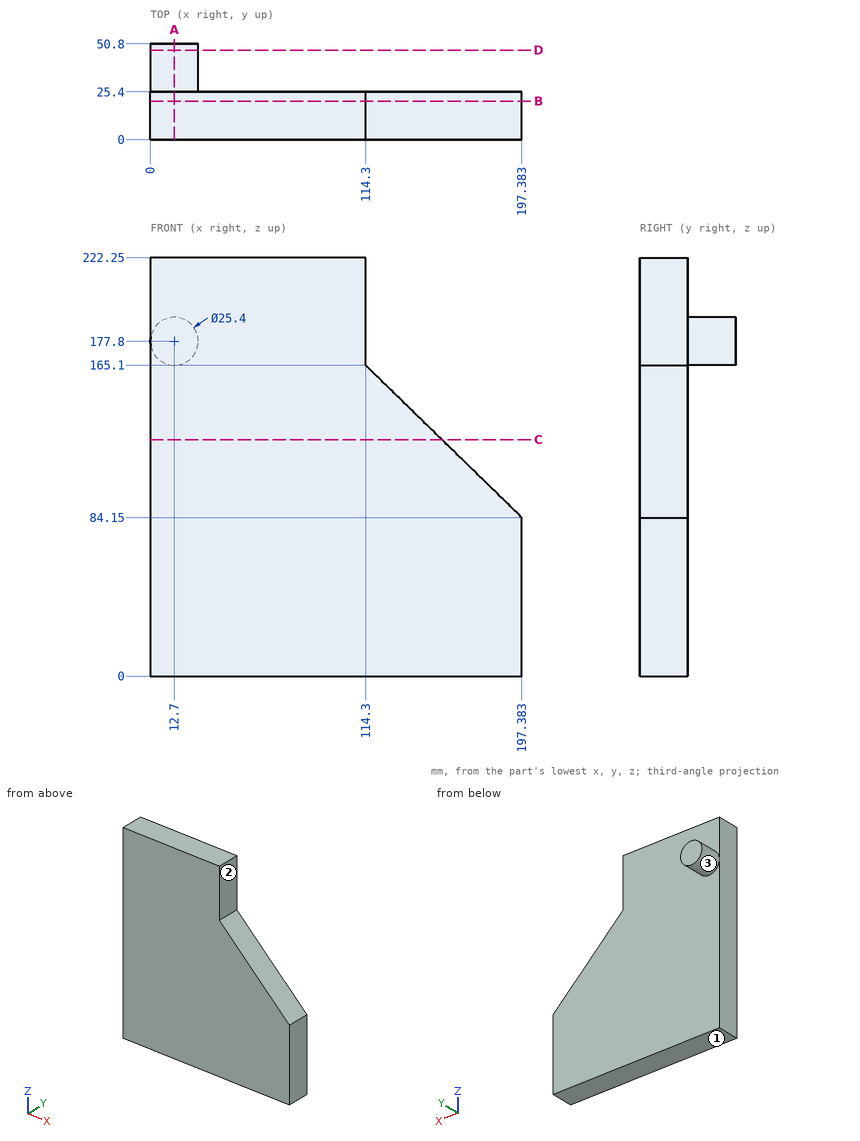
Answer from the drawing. Dimensions are ordinates in mm from the lowest x, y and z of the part. A direction names the side the tool comes from. Coordinates: 2 decimals unless noted, no trailing zeros. Order: outer loops, then holes, each group sorted by start corner. A loop starts at its lowest first (then second) coordinate and runs counter-clockwise, first axis right, second up. Notation, with made-up numbers: (79, 80.25) - (123, 80.25) arc R18 cw to (123, 110.25) - close; hole circle Ø3 at (-11.5, -13). An arc over 180 degrees is marked (long way). Put each result on its own line as item: value. Start each with the question number.
1) Find section D-D (y = 47.5). Give the vertices of the cut face in (x, z), plus the area to 3 significant figures.
2) Flat-ended cylindrical pins translate along their axes: pin 1 (20.5 mm diameter, centred on y = 14.5, z = 195.5, fed in from +X); pin 2 (10 mm diameter, centred on x = 116, z = 65.5, fed in from +Y); pin 3 (8 mm diameter, centred on x = 150, y = 8, fed in from +Z) (1 decimal). Find the tip coordinate at first contact, or state that the pin passes through.
3) Find section B-B (y = 20.5). Give the vertices of the cut face in (x, z).
4) Find section C-C (z = 125.5). Give the vertices of the cut face in (x, y), plus the area to 3 significant figures.
5) For the marked faces 1, 2 and 3, determine the directions among +Z, -Z, +X, -X, +Y, -Y from which every point of the face is accessible in a straight line to the end or side of a thin tool.
6) Find the intervals of material crossed by line 1 (Y direction, x = 101, z = 58.5); line 2 (X direction, y = 4, z = 187), in increasing order. Write a range as from..to.
7) Find section A-A (x = 12.7). Give the vertices of the cut face in (y, z), plus the area to 3 significant figures.
Results list:
1. outline: circle Ø25.4 at (12.7, 177.8)
1. area: 507 mm^2
2. pin 1: stops at x = 114.3
2. pin 2: stops at y = 25.4
2. pin 3: stops at z = 134.2
3. outline: (0, 0) - (197.38, 0) - (197.38, 84.15) - (114.3, 165.1) - (114.3, 222.25) - (0, 222.25) - close
4. outline: (0, 0) - (154.94, 0) - (154.94, 25.4) - (0, 25.4) - close
4. area: 3,940 mm^2
5. face 1: -Z, +X, -X, +Y, -Y
5. face 2: +Z, +X, +Y, -Y
5. face 3: +Y
6. line 1: y = 0..25.4
6. line 2: x = 0..114.3
7. outline: (0, 0) - (25.4, 0) - (25.4, 165.1) - (50.8, 165.1) - (50.8, 190.5) - (25.4, 190.5) - (25.4, 222.25) - (0, 222.25) - close
7. area: 6,290 mm^2
